from build123d import *

# Parameters (mm, degrees)
SKETCH1_R           = 18
SKETCH1_R_2         = 16.4
BOSS_EXTRUDE1_DEPTH = 6.4
SKETCH2_R           = 16.4
BOSS_EXTRUDE2_DEPTH = 1.2
SKETCH3_W           = 28.944907734
SKETCH3_H           = 19.372936664
SKETCH3_W_2         = 25.830582219
CUT_EXTRUDE1_DEPTH  = 9.2
SKETCH4_W           = 21.729498485
SKETCH4_H           = 20.961841185
CUT_EXTRUDE2_DEPTH  = 9.2
BOSS_EXTRUDE3_DEPTH = 4.2


with BuildPart() as part:
    # Sketch1 → Boss-Extrude1 (new body)
    with BuildSketch(Plane(origin=(0, 0, 0), x_dir=(1, 0, 0), z_dir=(0, 1, 0))):
        Circle(SKETCH1_R)
        Circle(SKETCH1_R_2, mode=Mode.SUBTRACT)
    extrude(amount=BOSS_EXTRUDE1_DEPTH)

    # Sketch2 → Boss-Extrude2 (add)
    with BuildSketch(Plane(origin=(0, 6.4, 0), x_dir=(1, 0, 0), z_dir=(0, 1, 0))):
        Circle(SKETCH2_R)
    extrude(amount=-BOSS_EXTRUDE2_DEPTH)

    # Sketch3 → Cut-Extrude1 (cut)
    with BuildSketch(Plane(origin=(0, 6.4, 0), x_dir=(1, 0, 0), z_dir=(0, 1, 0))):
        with Locations((-14.472453867, 9.686468332)):
            Rectangle(SKETCH3_W, SKETCH3_H)
        with Locations((12.91529111, 9.686468332)):
            Rectangle(SKETCH3_W_2, SKETCH3_H)
    extrude(amount=-CUT_EXTRUDE1_DEPTH, mode=Mode.SUBTRACT)

    # Sketch4 → Cut-Extrude2 (cut)
    with BuildSketch(Plane(origin=(0, 6.4, 0), x_dir=(1, 0, 0), z_dir=(0, 1, 0))):
        with Locations((10.864749243, -10.480920593)):
            Rectangle(SKETCH4_W, SKETCH4_H)
    extrude(amount=-CUT_EXTRUDE2_DEPTH, mode=Mode.SUBTRACT)

    # Sketch7 → Boss-Extrude3 (add)
    with BuildSketch(Plane.XZ):
        with BuildLine():
            Line((-7.071454056, 22.094943573), (0, 22.094943573))
            Line((0, 22.094943573), (0, 23))
            Line((0, 23), (-8.102673091, 23))
            add(Edge.make_bspline(
                [(-13.608541935, 11.781663143), (-11.344094103, 15.333566486), (-9.508804488, 19.073012106), (-8.102673091, 23)],
                knots=[0.222401663, 0.222401663, 0.222401663, 0.222401663, 0.927765661, 0.927765661, 0.927765661, 0.927765661], degree=3))
            ThreePointArc((-13.608541935, 11.781663143), (-12.071131769, 13.352444638), (-10.353735644, 14.724135228))
            add(Edge.make_bspline(
                [(-10.353735644, 14.724135228), (-9.080392431, 17.10273932), (-7.986298568, 19.559675436), (-7.071454056, 22.094943573)],
                knots=[0.464158141, 0.464158141, 0.464158141, 0.464158141, 0.920020117, 0.920020117, 0.920020117, 0.920020117], degree=3))
        make_face()
    extrude(amount=-BOSS_EXTRUDE3_DEPTH)


solid = part.part
Check sheet for the modelled part. Datum: model origin and axes. Units: mm. A direction names the side the tool comes from. Round coordinates to 2 decimals unless told otherwise and drop trailing zeros. Loops run counter-clockwise (first coordinate to the right, second up) from the corner with the lowest first, then second, coordinate; pieces in that order, holes last. Notation, with made-up numbers: (54.5, -26.75) -> (84.5, -26.75) arc R20 ccw to (84.5, 8.25) -> close; hole circle Ø5 at (37, 15). An arc over 180 degrees is marked (long way). Put each result on its own line as item: value. Start each with the question number.
1. Section check B-B (z = 6). Enter the section's corners in (x, y), plus the area to 3 significant figures.
2. Scan lines: probe 1 along Y at (x, z) = (-3.75, 4.5); probe 2 along Z at (x, y) = (-8, 1.25); probe 3 along Y at (x, z) = (-8.75, 19.25). Record each from-to range of solid material in increasing order.
3. Section check D-D (x = -14). Enter the section's corners in (y, z).
4. Section check A-A (x = -3.75). Enter the section's corners in (y, z).
5. Gauge pin test, flat ends, axial feed: pin 1 (1.5 mm diameter, centred on x = -15, y = 4.5, fed in from +Z); pin 2 (1.3 mm diameter, centred on x = -4.5, y = 1, fed in from -Z); pin 3 (2 mm diameter, centred on x = -6, y = 5.5, fed in from +Z). Record the tip position at first contact, or that the pin passes through.
6. Section check C-C (y = 4.75). Enter the section's corners in (x, z).
7. Access from +Z, -Z, +X, -X, +Y, -Y to the whole of each face (thin tool, end or side, straight path). Record for faces 1 (the face through (-11.72, 2.56, 11.47)), 2 (the face through (-4, 2, 22.095)), 3 (the face through (-7, 6.4, 7)), 4 (the face through (-8.3, 4.2, 19.5)).
Findings:
1. outline: (-16.97, 0) -> (-15.26, 0) -> (-15.26, 5.2) -> (0, 5.2) -> (0, 6.4) -> (-16.97, 6.4) -> close
1. area: 29.2 mm^2
2. probe 1: y = 5.2 to 6.4
2. probe 2: z = 14.32 to 16.12, 19.7 to 23
2. probe 3: y = 0 to 4.2
3. outline: (0, 8.54) -> (5.2, 8.54) -> (5.2, 0) -> (6.4, 0) -> (6.4, 11.31) -> (0, 11.31) -> close
4. outline: (0, 15.97) -> (5.2, 15.97) -> (5.2, 0) -> (6.4, 0) -> (6.4, 17.61) -> (0, 17.61) -> close; (0, 22.09) -> (4.2, 22.09) -> (4.2, 23) -> (0, 23) -> close
5. pin 1: stops at z = 11
5. pin 2: stops at z = 15.57
5. pin 3: stops at z = 17.29
6. outline: (-18, 0) -> (-16.4, 0) arc R16.4 cw to (0, 16.4) -> (0, 18) arc R18 ccw to start
7. face 1: -Z, +X, -Y
7. face 2: +X, +Y, -Y
7. face 3: +Z, -Z, +X, -X, +Y
7. face 4: +Z, -X, +Y
